from build123d import *

# Parameters (mm, degrees)
F0_R     = 9
F1_DEPTH = 50
F2_R     = 6
F3_R     = 0.5
F4_DEPTH = 25


with BuildPart() as f1:
    # F0 (on Right) → F1 (new body)
    with BuildSketch(Plane.YZ):
        Circle(F0_R)
    extrude(amount=F1_DEPTH)

    # F2
    f2_edges = [f1.edges().sort_by_distance(p)[0] for p in [
        (50, -9, 0),
        (0, -9, 0),
    ]]
    fillet(f2_edges, radius=F2_R)

    # F3 (on Top) → F4 (cut)
    with BuildSketch(Plane.XY):
        with Locations((8, 0)):
            Circle(F3_R)
    extrude(amount=F4_DEPTH, mode=Mode.SUBTRACT)


solid = f1.part
Part model, mm, in its own coordinate system. A direction names the side the tool comes from. Coordinates: 2 decimals unless noted, no trailing zeros. Write each loop counter-clockwise with the first axis right and the second up, starting at its lowest first coordinate (ties: lowest second). Pieces come first, ordered by that corner, then holes. Notation, with made-up numbers: (44, 46) - (55, 46) arc R15 cw to (55, 50) - close; hole circle Ø8 at (78.25, 25). An arc over 180 degrees is marked (long way). Put each result on its own line as item: value.
1. 3-axis set-ups, long thin cutter, end or side, ignore diameter. For faces 4 (the cylindrical face through (24.734, -1.172, 8.923)), 5 (the flat face through (8, 0, 0)): which of +Z, -Z, +X, -X, +Y, -Y reach the whole face in a straight line?
Final values:
face 4: +X, -X
face 5: +Z
2. Flat gauge pins, fed straight in: pin 1 Ø3 at (y, z) = (0, 6.5) entering from +X; pin 2 Ø1 at (x, y) = (26.5, 3.5) entering from +Z; pin 3 Ø5 at (x, z) = (23, -6.5) entering from +Y. Where does each tip first touch, or does it go through?
Final values:
pin 1: stops at x = 49.66
pin 2: stops at z = 8.49
pin 3: stops at y = 8.06
3. Two-plate mould, pull along X, no slides. Class faces 1 (the flat face through (50, 0, 0)), 2 (the cylindrical face through (8.462, -0.192, 4.437)), 3 (the flat face through (0, 0, 0)): +X half, -X half, draft (parallel to the pull), parting line (faces both ways), or undercut.
Final values:
face 1: +X half
face 2: undercut
face 3: -X half
4. Probe line 1 along X through (y, z) = (0, 7.25); line 2 along Y through (x, z) = (8, 2); line 3 along Y through (x, z) = (8, 6.75). List the from-to ranges inside material, lowest first. Write a range as [from, to].
Final values:
line 1: x = [1.76, 7.5], [8.5, 48.24]
line 2: y = [-8.77, -0.5], [0.5, 8.77]
line 3: y = [-5.95, -0.5], [0.5, 5.95]
5. Band-saw the part on B-B (x = 8). Write the cut outline in (y, z), then the cut area to 3 significant figures.
Final values:
outline: (-0.5, 0) - (-0.5, 8.99) arc R9 ccw (long way) to (0.5, 8.99) - (0.5, 0) - close
area: 245 mm²
6. Band-saw the part on A-A (x = 38.5). Write the cut outline in (y, z).
Final values:
outline: circle Ø18 at (0, 0)
